```python
from build123d import *

# Parameters (mm, degrees)
F0_R        = 152.4
F1_DEPTH    = 50.8
F2_R        = 103.4812283395
F3_DEPTH    = 63.5
F5_R        = 152.1778472169
F6_DEPTH    = 50.8
F7_S5_R     = 103.4812283395
F7_T6_DEPTH = 218
F8_S5_R     = 103.4812283395
F8_T6_DEPTH = 219
F9_R        = 25.5370078958
F10_DEPTH   = 203.2


# Not quite as in the source:
# - a fillet or chamfer that OpenCascade refuses, or shapes differently, is made with other operations: its cross-section is extruded or revolved along the edge and cut away or added


with BuildPart() as f1:
    # F0 (on Top) → F1 (new body)
    with BuildSketch(Plane.XY):
        Circle(F0_R)
    extrude(amount=F1_DEPTH)

    # F2 (on face) → F3 (join)
    with BuildSketch(Plane.XY.offset(50.8)):
        Circle(F2_R)
    extrude(amount=F3_DEPTH)

    # F5 (on face) → F6 (join)
    with BuildSketch(Plane.XY.offset(114.3)):
        Circle(F5_R)
    extrude(amount=F6_DEPTH)

    # F7: chamfer of 50.8 on 1 edges, made by hand


with BuildPart() as f7_tool2:
    # F7_s3 → F7_t4 (revolve)
    with BuildSketch(Plane.XZ):
        Polygon((152.1778472169, 165.1), (101.3778472169, 114.3), (152.1778472169, 114.3), align=None)
    revolve(axis=Axis((0, 0, 114.3), (0, 0, 1)))

    # F7_s5 → F7_t6 (cut, symmetric)
    with BuildSketch(Plane.XY.offset(139.7)):
        Circle(F7_S5_R)
    extrude(amount=F7_T6_DEPTH, both=True, mode=Mode.SUBTRACT)


with BuildPart() as f1_1:
    add(f1.part)

    # F7_t1: cut F7_tool2
    add(f7_tool2.part, mode=Mode.SUBTRACT)

    # F8: chamfer of 50.8 on 1 edges, made by hand


with BuildPart() as f8_tool2:
    # F8_s3 → F8_t4 (revolve)
    with BuildSketch(Plane.XZ):
        Polygon((101.6, 50.8), (152.4, 0), (152.4, 50.8), align=None)
    revolve(axis=Axis((0, 0, 50.8), (0, 0, 1)))

    # F8_s5 → F8_t6 (cut, symmetric)
    with BuildSketch(Plane.XY.offset(25.4)):
        Circle(F8_S5_R)
    extrude(amount=F8_T6_DEPTH, both=True, mode=Mode.SUBTRACT)


with BuildPart() as f1_2:
    add(f1_1.part)

    # F8_t1: cut F8_tool2
    add(f8_tool2.part, mode=Mode.SUBTRACT)

    # F9 (on face) → F10 (cut)
    with BuildSketch(Plane.XY.offset(165.1)):
        Circle(F9_R)
    extrude(amount=-F10_DEPTH, mode=Mode.SUBTRACT)


solid = f1_2.part
```
Check sheet for the modelled part. Datum: model origin and axes. Units: mm. A direction names the side the tool comes from. Give positions to 0.01 mm unless a question says otherwise; leave off trailing zeros. Write each loop counter-clockwise with the first axis right and the second up, starting at its lowest first coordinate (ties: lowest second). Pieces come first, ordered by that corner, then holes. Notation, with made-up numbers: (14.5, -24) - (36.5, -24) arc R27 ccw to (36.5, -1) - close; hole circle Ø8 at (3.5, 44.5). An arc over 180 degrees is marked (long way). Answer as a JSON object with one key per item and string values. Group by question number.
1) Access from +Z, -Z, +X, -X, +Y, -Y to the whole of each face (thin tool, end or side, straight path). Record for faces 4 (the face through (97.775, -40.54, 118.768)), 5 (the face through (13.73, 21.53, 83.71)).
2) Release check for a two-part mould opening along Z. For faces 1 (the face through (-2, -32, 165.1)), 2 (the face through (101.62, 32, 45.86)), 3 (the face through (32, 2, 0)) record: pulls with the +Z half, pulls with the -Z half, needs draft (parallel to the pull), parting line crosses it, or undercut.
3) Sectioned sample at D-D (z = 149). Record the cut outline in (x, y).
4) Thickness scan on probe 1 along Y at (x, z) = (0, 64); probe 2 along Y at (x, z) = (0, 128); probe 3 along Z at (x, y) = (77.5, 88). Record the ranges inside material, lowest first. Write a range as from..to.
5) Sectioned sample at C-C (z = 99.5). Record the cut outline in (x, y), then the cut area to 3 significant figures.
6) Sectioned sample at A-A (x = 0). Record the cut outline in (y, z).
7) Depth check by flat-ended pin: P1, Ø2, axis at y = -71.5, z = 84, coming from the +X side; P2, Ø6, axis at y = 23, z = 24, coming from the -X side; P3, Ø6, axis at y = 57.5, z = 63, coming from the +X side. Enter the tip coordinate at first touch or a pass-through.
Geometry results:
{
 "1": {"face 4": "none", "face 5": "+Z, -Z"},
 "2": {"face 1": "pulls with the +Z half", "face 2": "undercut", "face 3": "pulls with the -Z half"},
 "3": {"outline": "circle Ø272.16 at (0, 0); hole circle Ø51.07 at (0, 0)"},
 "4": {"probe 1": "y = -103.48..-25.54, 25.54..103.48", "probe 2": "y = -115.08..-25.54, 25.54..115.08", "probe 3": "z = 0..35.14, 130.18..165.1"},
 "5": {"outline": "circle Ø206.96 at (0, 0); hole circle Ø51.07 at (0, 0)", "area": "31,600 mm^2"},
 "6": {"outline": "(-152.4, 0) - (-25.54, 0) - (-25.54, 165.1) - (-152.18, 165.1) - (-103.48, 116.4) - (-103.48, 48.92) - close; (25.54, 0) - (152.4, 0) - (103.48, 48.92) - (103.48, 116.4) - (152.18, 165.1) - (25.54, 165.1) - close"},
 "7": {"P1": "stops at x = 75.75", "P2": "stops at x = -129.42", "P3": "stops at x = 87.97"}
}
